Design review of the part built by this model. Coordinates are the model's own, in mm. Round coordinates to 2 decimals unless told otherwise and drop trailing zeros. Order: outer loops, then holes, each group sorted by start corner. A loop starts at its lowest first (then second) coordinate and runs counter-clockwise, first axis right, second up.
from build123d import *


with BuildPart() as part:
    # Sketch1 → Revolve1 (revolve)
    with BuildSketch(Plane.XY):
        with BuildLine():
            Line((8.94427191, 37), (15.5, 37))
            Line((15.5, 37), (15.5, 27.1))
            ThreePointArc((15.5, 27.1), (14.88492424, 25.61507576), (13.4, 25))
            Line((13.4, 25), (-13.4, 25))
            ThreePointArc((-13.4, 25), (-14.88492424, 25.61507576), (-15.5, 27.1))
            Line((-15.5, 27.1), (-15.5, 37))
            Line((-15.5, 37), (-8.94427191, 37))
            ThreePointArc((-8.94427191, 37), (0, 33), (8.94427191, 37))
        make_face()
    revolve(axis=Axis((-44.328053157, 0, 0), (1, 0, 0)))


solid = part.part
1) Take a section at A-A on z = 0. Give the boundary of the cut face in (x, y), plus the area to 3 significant figures.
Results:
outline: (-15.5, -37) - (-8.94, -37) arc R12 cw to (8.94, -37) - (15.5, -37) - (15.5, -27.1) arc R2.1 ccw to (13.4, -25) - (-13.4, -25) arc R2.1 ccw to (-15.5, -27.1) - close; (-15.5, 27.1) arc R2.1 ccw to (-13.4, 25) - (13.4, 25) arc R2.1 ccw to (15.5, 27.1) - (15.5, 37) - (8.94, 37) arc R12 cw to (-8.94, 37) - (-15.5, 37) - close
area: 641 mm2
2) Take a section at D-D on x = 0.5. Give the boundary of the cut face in (y, z), plus the area to 3 significant figures.
Results:
outline: circle Ø66.02 at (0, 0); hole circle Ø50 at (0, 0)
area: 1,460 mm2
3) Clearance check with flat-ended pins moving along their axes: P1, Ø3, axis at x = -12.5, z = 12, coming from the -Y side; P2, Ø4, axis at x = -10, y = 19, coming from the +Z side; P3, Ø3, axis at x = -2.5, y = 8.5, coming from the -Z side; P4, Ø1, axis at y = 11.5, z = 21, coming from the -X side. State where each tip first meets the part, or that it passes through.
Results:
P1: stops at y = -35.48
P2: stops at z = 32.86
P3: stops at z = -32.71
P4: passes through
4) To check wall thickness, follow line 1 along Z through (x, y) = (-6, 1.5); line 2 along Z through (x, y) = (3, 20); line 3 along Y through (x, z) = (0.5, -1.5). State the ranges of each line that lie inside material, in increasing order.
Results:
line 1: z = -34.58 to -24.95, 24.95 to 34.58
line 2: z = -26.73 to -15, 15 to 26.73
line 3: y = -32.98 to -24.95, 24.95 to 32.98
5) Take a section at C-C on x = -11. Give the boundary of the cut face in (y, z), plus the area to 3 significant figures.
Results:
outline: circle Ø74 at (0, 0); hole circle Ø50 at (0, 0)
area: 2,340 mm2
6) The part is to be moulded in two halves that separate along Y. For faces 1 (the face through (12.27, -8.02, -36.12)), 2 (the face through (-0.188, 23.846, 7.509)), 3 (the face through (-15.5, 19.4, 19.4)), say which applies: released by +Y, released by -Y, zero draft, split by the parting line, or undercut.
Results:
face 1: split by the parting line
face 2: undercut
face 3: zero draft
